CAD build for the part. Positions are in the model's coordinates, mm. Face numbers are marked on the shaded views. Round coordinates to 2 decimals unless told otherwise and drop trailing zeros. Loops run counter-clockwise (first coordinate to the right, second up) from the corner with the lowest first, then second, coordinate; pieces in that order, holes last.
from build123d import *

# Parameters (mm, degrees)
BOSS_EXTRUDE1_DEPTH   = 2.5
BOSS_EXTRUDE1_2_DEPTH = 2.5
BOSS_EXTRUDE1_3_DEPTH = 2.5
BOSS_EXTRUDE1_4_DEPTH = 2.5
SKETCH1_3_R           = 12.5
SKETCH1_3_R_2         = 10.25
BOSS_EXTRUDE2_DEPTH   = 80


with BuildPart() as part:
    # Sketch1 → Boss-Extrude1 (new body)
    with BuildSketch(Plane(origin=(0, 0, 0), x_dir=(1, 0, 0), z_dir=(0, 1, 0))):
        with BuildLine():
            ThreePointArc((-1.4, 12.421352583), (0, 12.5), (1.4, 12.421352583))
            Line((1.4, 12.421352583), (1.4, 14.934523762))
            ThreePointArc((1.4, 14.934523762), (0, 15), (-1.4, 14.934523762))
            Line((-1.4, 14.934523762), (-1.4, 12.421352583))
        make_face()
    extrude(amount=-BOSS_EXTRUDE1_DEPTH)



with BuildPart() as body_2:
    # Sketch1 → Boss-Extrude1 2 (new body)
    with BuildSketch(Plane(origin=(0, 0, 0), x_dir=(1, 0, 0), z_dir=(0, 1, 0))):
        with BuildLine():
            Line((14.934523762, 1.4), (12.421352583, 1.4))
            ThreePointArc((12.421352583, 1.4), (12.480322658, 0.701103669), (12.5, 0))
            ThreePointArc((12.5, 0), (12.480322658, -0.701103669), (12.421352583, -1.4))
            Line((12.421352583, -1.4), (14.934523762, -1.4))
            ThreePointArc((14.934523762, -1.4), (14.983621999, -0.700765142), (15, 0))
            ThreePointArc((15, 0), (14.983621999, 0.700765142), (14.934523762, 1.4))
        make_face()
    extrude(amount=-BOSS_EXTRUDE1_2_DEPTH)


with BuildPart() as body_3:
    # Sketch1 → Boss-Extrude1 3 (new body)
    with BuildSketch(Plane(origin=(0, 0, 0), x_dir=(1, 0, 0), z_dir=(0, 1, 0))):
        with BuildLine():
            ThreePointArc((-12.421352583, -1.4), (-12.5, 0), (-12.421352583, 1.4))
            Line((-12.421352583, 1.4), (-14.934523762, 1.4))
            ThreePointArc((-14.934523762, 1.4), (-15, 0), (-14.934523762, -1.4))
            Line((-14.934523762, -1.4), (-12.421352583, -1.4))
        make_face()
    extrude(amount=-BOSS_EXTRUDE1_3_DEPTH)


with BuildPart() as body_4:
    # Sketch1 → Boss-Extrude1 4 (new body)
    with BuildSketch(Plane(origin=(0, 0, 0), x_dir=(1, 0, 0), z_dir=(0, 1, 0))):
        with BuildLine():
            Line((1.4, -14.934523762), (1.4, -12.421352583))
            ThreePointArc((1.4, -12.421352583), (0, -12.5), (-1.4, -12.421352583))
            Line((-1.4, -12.421352583), (-1.4, -14.934523762))
            ThreePointArc((-1.4, -14.934523762), (0, -15), (1.4, -14.934523762))
        make_face()
    extrude(amount=-BOSS_EXTRUDE1_4_DEPTH)


with BuildPart() as part_1:
    add(part.part)

    add(body_2.part)  # Boss-Extrude2 merges body 2

    add(body_3.part)  # Boss-Extrude2 merges body 3

    add(body_4.part)  # Boss-Extrude2 merges body 4
    # Sketch1_3 → Boss-Extrude2 (add)
    with BuildSketch(Plane(origin=(0, 0, 0), x_dir=(1, 0, 0), z_dir=(0, 1, 0))):
        with Locations(Location((0, 0, 0), (0, 0, 270))):
            Circle(SKETCH1_3_R)
        with Locations(Location((0, 0, 0), (0, 0, 270))):
            Circle(SKETCH1_3_R_2, mode=Mode.SUBTRACT)
    extrude(amount=-BOSS_EXTRUDE2_DEPTH)


solid = part_1.part
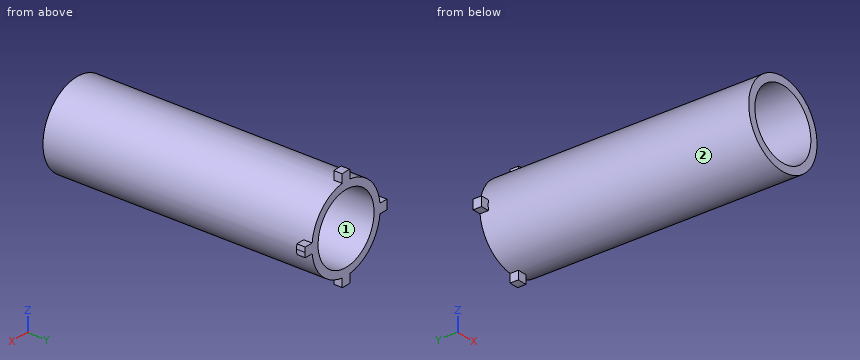
Item 1: Mould opens along X. For the marked faces 1 and 2 say: released by +X, released by -X, zero draft, split by the parting line, or undercut.
Verdict:
face 1: undercut
face 2: split by the parting line
Item 2: Cut at D-D (x = -7.5). List the corners of the cut face in (y, z).
Verdict:
outline: (-80, -10) - (0, -10) - (0, -6.99) - (-80, -6.99) - close; (-80, 6.99) - (0, 6.99) - (0, 10) - (-80, 10) - close
Item 3: Cut at C-C (y = -36). List the corners of the cut face in (x, z), plus the area to 3 significant figures.
Verdict:
outline: circle Ø25 at (0, 0); hole circle Ø20.5 at (0, 0)
area: 161 mm2
Item 4: Wall check: L1, parallel to X at y = -44, z = 0; L2, parallel to X at y = -28, z = -8.25; L3, parallel to Z at x = -1.5, y = -7.5. Give the ranges that are in metal, low to high.
Verdict:
L1: x = -12.5 to -10.25, 10.25 to 12.5
L2: x = -9.39 to -6.08, 6.08 to 9.39
L3: z = -12.41 to -10.14, 10.14 to 12.41
Item 5: Cut at B-B (z = -9.25). List the corners of the cut face in (x, y), plus the area to 3 significant figures.
Verdict:
outline: (-8.41, -80) - (-4.42, -80) - (-4.42, 0) - (-8.41, 0) - close; (4.42, -80) - (8.41, -80) - (8.41, 0) - (4.42, 0) - close
area: 639 mm2
Item 6: Flat gauge pins, fed straight in: P1, Ø0.8, axis at y = -1.5, z = -14, coming from the +X side; P2, Ø2, axis at x = -2.5, y = -22, coming from the -Z side; P3, Ø1.2, axis at x = 13.5, y = -1.5, coming from the -Z side; P4, Ø10, axis at x = 2, z = -8, coming from the -Y side. Where does each tip first touch, or does it go through?
Verdict:
P1: stops at x = 1.4
P2: stops at z = -12.41
P3: stops at z = -1.4
P4: stops at y = -80
Item 7: Cut at A-A (x = 0). List the corners of the cut face in (y, z), plus the area to 4 significant figures.
Verdict:
outline: (-80, -12.5) - (-2.5, -12.5) - (-2.5, -15) - (0, -15) - (0, -10.25) - (-80, -10.25) - close; (-80, 10.25) - (0, 10.25) - (0, 15) - (-2.5, 15) - (-2.5, 12.5) - (-80, 12.5) - close
area: 372.5 mm2
